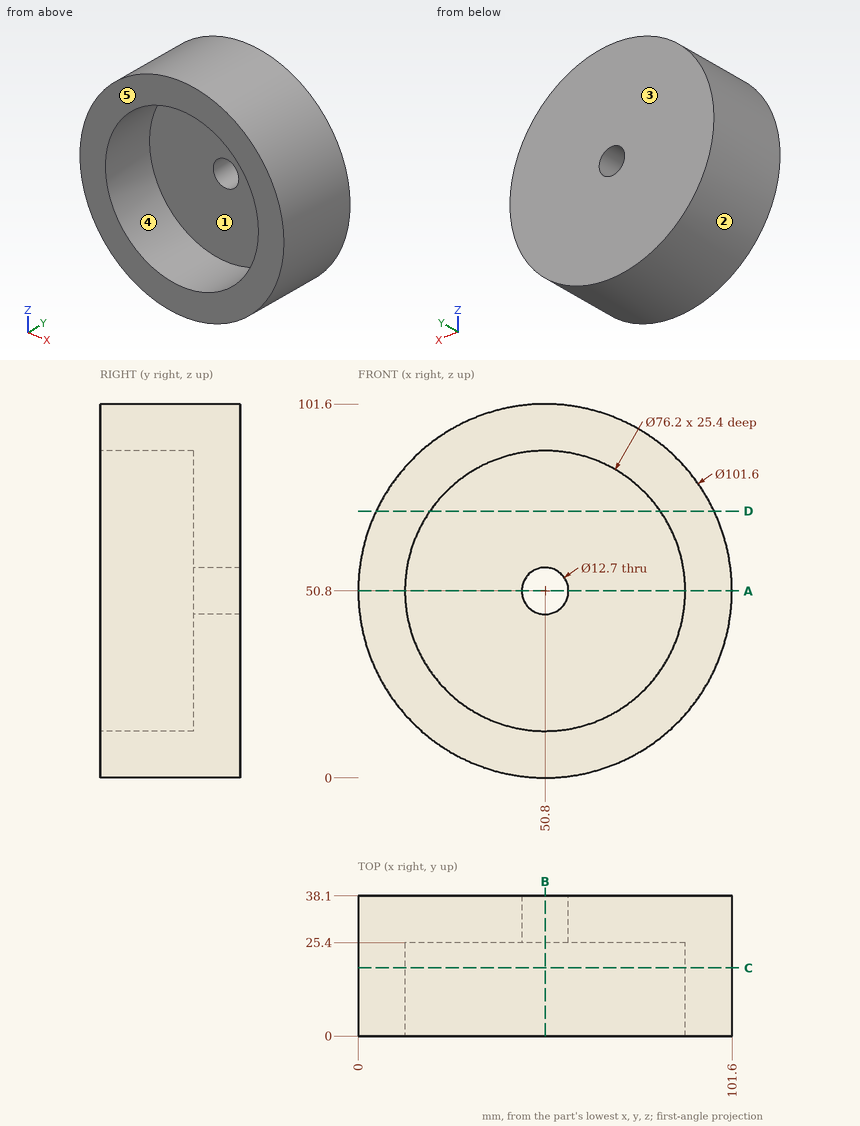
The figure shows three views and two pictorial views of one solid part (mm, origin at its lowest corner). Answer the questions. A direction names the side the tool comes from. Give positions to 0.01 mm unless a question says otherwise; leave off trailing zeros. Write each loop counter-clockwise with the first axis right and the second up, starting at its lowest first coordinate (ties: lowest second). Pieces come first, ordered by that corner, then holes. Notation, with made-up numbers: (65, 39.5) - (121, 39.5) arc R31 ccw to (121, 70.5) - close; hole circle Ø5 at (26, -15.5). An arc over 180 degrees is marked (long way). Return JSON: item names as keys, results as strings.
Q1. A cutting plane is placed at D-D, the plane z = 72.5. Determine the outline of the cut face in (x, y).
Reply:
{"outline": "(4.87, 0) - (19.48, 0) - (19.48, 25.4) - (82.12, 25.4) - (82.12, 0) - (96.73, 0) - (96.73, 38.1) - (4.87, 38.1) - close"}
Q2. Given P1, Ø5, axis at x = 74.5, z = 57, coming from the -Y side; P2, Ø10, axis at y = 26, z = 14, coming from the -X side; P3, Ø10, axis at y = 15.5, z = 46, coming from the +X side; P4, Ø6, axis at x = 12.5, y = 25.5, coming from the +Z side, each flat-ended and moving along its own axis, determine where each tip first touches the part or whether it passes through.
Reply:
{"P1": "y = 25.4", "P2": "x = 11.18", "P3": "x = 101.6", "P4": "z = 87.33"}
Q3. For a pull along X with two mould halves and no side action, classify the marked faces 1, 2 and 3 as released by +X, released by -X, zero draft, split by the parting line, or undercut.
Reply:
{"face 1": "undercut", "face 2": "split by the parting line", "face 3": "zero draft"}
Q4. A cutting plane is placed at C-C, the plane y = 18.5. Determine the outline of the cut face in (x, z), and give its area (3 significant figures).
Reply:
{"outline": "circle Ø101.6 at (50.8, 50.8); hole circle Ø76.2 at (50.8, 50.8)", "area": "3,550 mm²"}
Q5. Consider line 1 along Z through (x, y) = (50.8, 33); line 2 along Z through (x, y) = (50.8, 15.5); line 3 along Y through (x, z) = (78, 30.5). Determine where each line is inside the solid, lowest interval first. Write a range as [from, to].
Reply:
{"line 1": "[0, 44.45], [57.15, 101.6]", "line 2": "[0, 12.7], [88.9, 101.6]", "line 3": "[25.4, 38.1]"}
Q6. For the marked faces 4 and 5, determine the directions among +Z, -Z, +X, -X, +Y, -Y from which every point of the face is accessible in a straight line to the end or side of a thin tool.
Reply:
{"face 4": "-Y", "face 5": "+Z, -Z, +X, -X, -Y"}
Q7. A cutting plane is placed at A-A, the plane z = 50.8. Determine the outline of the cut face in (x, y).
Reply:
{"outline": "(0, 0) - (12.7, 0) - (12.7, 25.4) - (44.45, 25.4) - (44.45, 38.1) - (0, 38.1) - close; (57.15, 25.4) - (88.9, 25.4) - (88.9, 0) - (101.6, 0) - (101.6, 38.1) - (57.15, 38.1) - close"}
Q8. A cutting plane is placed at B-B, the plane x = 50.8. Determine the outline of the cut face in (y, z), and give its area (3 significant figures).
Reply:
{"outline": "(0, 0) - (38.1, 0) - (38.1, 44.45) - (25.4, 44.45) - (25.4, 12.7) - (0, 12.7) - close; (0, 88.9) - (25.4, 88.9) - (25.4, 57.15) - (38.1, 57.15) - (38.1, 101.6) - (0, 101.6) - close", "area": "1,770 mm²"}
